Autodesk Inventor part; units mm, degrees
ref_plane "YZ Plane" through (0, 0, 0) normal (1, 0, 0) x (0, 1, 0)
ref_plane "XZ Plane" through (0, 0, 0) normal (0, 1, 0) x (-1, 0, 0)
ref_plane "XY Plane" through (0, 0, 0) normal (0, 0, 1) x (1, 0, 0)
sketch "Sketch1" plane through (0, 0, 0) normal (0, 1, 0) x (-1, 0, 0)
  circle A0 centre (0, 0) radius 18
  dimension "d0" = 36
extrude "Extrusion1" add sketch "Sketch1" along normal blind 2
sketch "Sketch2" plane through (0, 2, 0) normal (0, 1, 0) x (1, 0, 0)
  circle A0 centre (0, 0) radius 12
  circle A1 centre (0, 0) radius 14
  dimension "d5" = 24
  dimension "d6" = 28
extrude "Extrusion2" add sketch "Sketch2" along normal blind 14
sketch "Sketch3" plane through (0, 2, 0) normal (0, 1, 0) x (1, 0, 0)
  circle A0 centre (0, 0) radius 3
  dimension "d9" = 6
hole "Hole1" at (0, 2, 0) direction (0, -1, 0) diameter 6 end through all
sketch "Sketch4" plane through (0, 2, 0) normal (0, 1, 0) x (1, 0, 0)
  circle A0 centre (0, 0) radius 21
  dimension "d17" = 42
extrude "Extrusion3" add sketch "Sketch4" against normal blind 2
sketch "Sketch5" plane through (0, 2, 0) normal (0, 1, 0) x (1, 0, 0)
  point P0 (0, 0)
  point P1 (0, 0)
hole "Hole2" at (0, 2, 0) direction (0, -1, 0) diameter 6 end through all
properties part number "foot_bearings_holder" material "PET Plastic"
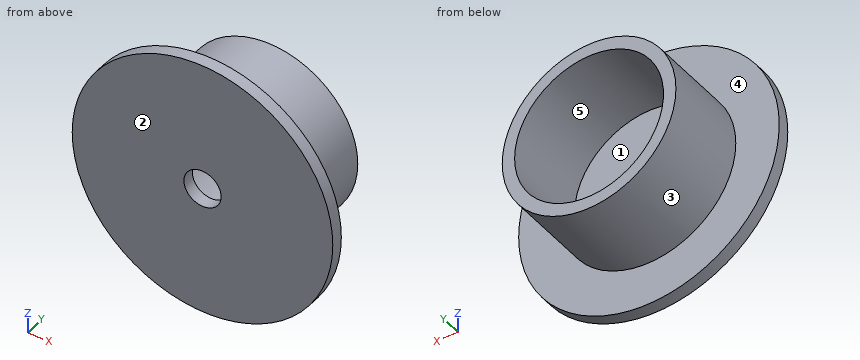
Geometry: final body of the model. Coordinates: model frame, mm. Face numbers are marked on the shaded views. A direction names the side the tool comes from. Round coordinates to 2 decimals unless told otherwise and drop trailing zeros. Order: outer loops, then holes, each group sorted by start corner. A loop starts at its lowest first (then second) coordinate and runs counter-clockwise, first axis right, second up. Notation, with made-up numbers: M 22.25,36.25 L 79.25,36.25 A30 ccw 79.25,61.25 Z; hole C 88.25,28.5 d7. An arc over 180 degrees is marked long. One line per item, written item: value.
(1) Cut plane B-B (x = 0). Return the cut outline in (y, z), and give its area (3 significant figures).
Result sheet:
outline: M 0,-21 L 2,-21 L 2,-14 L 16,-14 L 16,-12 L 2,-12 L 2,-3 L 0,-3 Z; M 0,3 L 2,3 L 2,12 L 16,12 L 16,14 L 2,14 L 2,21 L 0,21 Z
area: 128 mm2
(2) Cut plane C-C (x = 6). Return the cut outline in (y, z), and give its area (3 significant figures).
Result sheet:
outline: M 0,-20.12 L 2,-20.12 L 2,-12.65 L 16,-12.65 L 16,-10.39 L 2,-10.39 L 2,10.39 L 16,10.39 L 16,12.65 L 2,12.65 L 2,20.12 L 0,20.12 Z
area: 144 mm2
(3) Cut plane D-D (y = 12.75). Return the cut outline in (x, z).
Result sheet:
outline: C 0,0 d28; hole C 0,0 d24
(4) Reachability of the marked faces 1 and 2 from +Z, -Z, +X, -X, +Y, -Y: full face, straight path, thin tool, end or side. Return the list, or none.
Result sheet:
face 1: +Y
face 2: +Z, -Z, +X, -X, -Y
(5) Pin query (flat end, axial travel): P1, Ø10, axis at x = 16.5, z = 1, coming from the -Y side; P2, Ø6, axis at y = 8.5, z = 12.5, coming from the -X side; P3, Ø7, axis at x = 4, z = 5, coming from the +Y side; P4, Ø4, axis at x = 3, y = 14, coming from the +Z side. Return the tip coordinate at first contact, or that it passes through.
Result sheet:
P1: y = 0
P2: x = -10.28
P3: y = 2
P4: z = 13.96
(6) Pull-direction query (Z, two-part tool) for the marked faces 3, 4 and 5; classes: pulls with the +Z half, pulls with the -Z half, needs draft (parallel to the pull), parting line crosses it, or undercut.
Result sheet:
face 3: parting line crosses it
face 4: needs draft
face 5: undercut
(7) Cut plane A-A (z = 0). Return the cut outline in (x, y), and give its area (3 significant figures).
Result sheet:
outline: M -21,0 L -3,0 L -3,2 L -12,2 L -12,16 L -14,16 L -14,2 L -21,2 Z; M 3,0 L 21,0 L 21,2 L 14,2 L 14,16 L 12,16 L 12,2 L 3,2 Z
area: 128 mm2
(8) Line query: probe 1 along X at (y, z) = (1.1, 0); probe 2 along X at (y, z) = (5.75, 0). Output: solid intervals per line, ascending. Write a range as [from, to].
Result sheet:
probe 1: [-21, -3], [3, 21]
probe 2: [-14, -12], [12, 14]
